Geometry: final body of the model. Coordinates: model frame, mm. Face numbers are marked on the shaded views. A direction names the side the tool comes from. Round coordinates to 2 decimals unless told otherwise and drop trailing zeros. Loops run counter-clockwise (first coordinate to the right, second up) from the corner with the lowest first, then second, coordinate; pieces in that order, holes last. Notation, with made-up numbers: (-11, 47) - (4, 47) arc R16 cw to (4, 78) - close; hole circle Ø5 at (-5, 80.5). An arc over 180 degrees is marked (long way). Return JSON: item names as keys, results as strings. Group by question number.
1. Section A-A on z = 8. Return loops of the section in (x, y), and give its area (3 significant figures).
2. Set-up query: the marked faces 4 and 5. Return all of +Z, -Z, +X, -X, +Y, -Y with unobstructed straight access to the full face (end or side cutting, diameter ignored); none if empty.
3. Material intervals for probe 1 along X at (y, z) = (-0.25, 3.5); probe 2 along X at (y, z) = (-8.75, 2); probe 3 along Y at (x, z) = (6.5, 6.75), sorted ascending.
4. Section C-C on y = -3. Return loops of the section in (x, z).
5. Draft query along X for the marked faces 1, 2 and 3. Return one class per face: +X half, -X half, draft (parallel to the pull), parting line (faces both ways), or undercut.
6. Section D-D on y = -10. Return loops of the section in (x, z), and give its area (3 significant figures).
7. First-contact query: pin 1 Ø1.5 at (x, z) = (19, 10.5) entering from +Y; pin 2 Ø3 at (x, y) = (-10.5, -8) entering from +Z. Flat tips, straight axial feed; report the tip coordinate or a pass-through.
8. Section B-B on x = -17. Return loops of the section in (y, z), and give its area (3 significant figures).
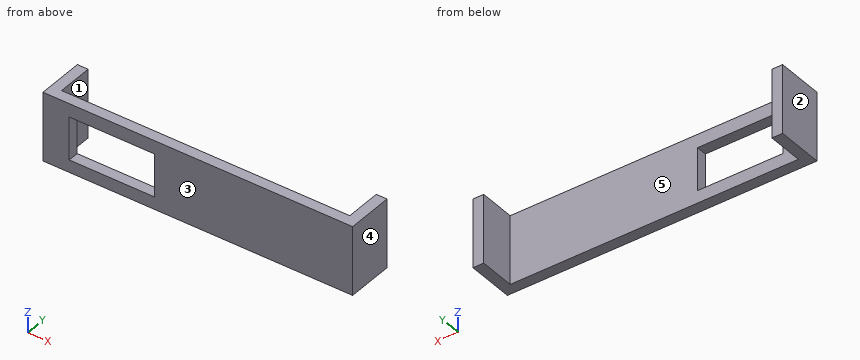
from build123d import *

# Parameters (mm, degrees)
F0_W     = 72.1
F0_H     = 16
F1_DEPTH = 10.9
F2_T     = -2.5
F3_W     = 19.88007
F3_H     = 10
F4_DEPTH = 25


with BuildPart() as f1:
    # F0 (on Front) → F1 (new body)
    with BuildSketch(Plane.XZ):
        with Locations((-0.508198, 5.101174)):
            Rectangle(F0_W, F0_H)
    extrude(amount=F1_DEPTH)

    # F2
    f2_openings = [f1.faces().sort_by_distance(p)[0] for p in [
        (-0.508198, 0, 5.101174),
        (-0.508198, -5.45, 13.101174),
        (-0.508198, -5.45, -2.898826),
    ]]
    offset(amount=F2_T, openings=f2_openings)

    # F3 (on face) → F4 (cut)
    with BuildSketch(Plane.XZ.offset(10.9)):
        with Locations((-20.508622, 5)):
            Rectangle(F3_W, F3_H)
    extrude(amount=-F4_DEPTH, mode=Mode.SUBTRACT)


solid = f1.part
Taken from the geometry:
{
 "1": {"outline": "(-36.56, -10.9) - (-30.45, -10.9) - (-30.45, -8.4) - (-34.06, -8.4) - (-34.06, 0) - (-36.56, 0) - close; (-10.57, -10.9) - (35.54, -10.9) - (35.54, 0) - (33.04, 0) - (33.04, -8.4) - (-10.57, -8.4) - close", "area": "173 mm2"},
 "2": {"face 4": "+Z, -Z, +X, +Y, -Y", "face 5": "+Z, -Z, +Y"},
 "3": {"probe 1": "-36.56 to -34.06, 33.04 to 35.54", "probe 2": "-36.56 to -30.45, -10.57 to 35.54", "probe 3": "-10.9 to -8.4"},
 "4": {"outline": "(-36.56, -2.9) - (-34.06, -2.9) - (-34.06, 13.1) - (-36.56, 13.1) - close; (33.04, -2.9) - (35.54, -2.9) - (35.54, 13.1) - (33.04, 13.1) - close"},
 "5": {"face 1": "undercut", "face 2": "-X half", "face 3": "draft"},
 "6": {"outline": "(-36.56, -2.9) - (35.54, -2.9) - (35.54, 13.1) - (-36.56, 13.1) - close; hole (-30.45, 0) - (-10.57, 0) - (-10.57, 10) - (-30.45, 10) - close", "area": "955 mm2"},
 "7": {"pin 1": "y = -8.4", "pin 2": "z = 13.1"},
 "8": {"outline": "(-10.9, -2.9) - (-8.4, -2.9) - (-8.4, 0) - (-10.9, 0) - close; (-10.9, 10) - (-8.4, 10) - (-8.4, 13.1) - (-10.9, 13.1) - close", "area": "15.0 mm2"}
}
